Autodesk Inventor part; units mm, degrees
ref_plane "YZ Plane" through (0, 0, 0) normal (1, 0, 0) x (0, 1, 0)
ref_plane "XZ Plane" through (0, 0, 0) normal (0, 1, 0) x (-1, 0, 0)
ref_plane "XY Plane" through (0, 0, 0) normal (0, 0, 1) x (1, 0, 0)
sketch "Sketch1" plane through (0, 0, 0) normal (0, 1, 0) x (-1, 0, 0)
  line L0 (0, 0) -> (-111, 0)
  line L1 (-111, 0) -> (-111, -34)
  line L2 (-111, -34) -> (0, -34)
  line L3 (0, -34) -> (0, 0)
  dimension "d0" = 111
  dimension "d1" = 34
extrude "Extrusion1" add sketch "Sketch1" along normal blind 3.5
sketch "Sketch2" plane through (0, 3.5, 0) normal (0, 1, 0) x (1, 0, 0)
  line L0 (10, 9.825) -> (40, 9.825)
  line L1 (40, 9.825) -> (40, 24.175)
  line L2 (40, 24.175) -> (10, 24.175)
  line L3 (10, 24.175) -> (10, 9.825)
  line L4 (66.65, 9.825) -> (96.65, 9.825)
  line L5 (96.65, 9.825) -> (96.65, 24.175)
  line L6 (96.65, 24.175) -> (66.65, 24.175)
  line L7 (66.65, 24.175) -> (66.65, 9.825)
  point P0 (0, 0)
  point P1 (66.65, 17)
  dimension "d4" = 30
  dimension "d5" = 14.35
  dimension "d6" = 30
  dimension "d7" = 14.35
  dimension "d8" = 26.65
extrude "Extrusion2" cut sketch "Sketch2" against normal blind 3.5
fillet "Fillet1" radius 2 8 edges at (10, 1.75, -24.175) (40, 1.75, -24.175) (10, 1.75, -9.825) (40, 1.75, -9.825) (66.65, 1.75, -9.825) (66.65, 1.75, -24.175) (96.65, 1.75, -9.825) (96.65, 1.75, -24.175)
properties part number "arcade_lid_extrusion_3.5"
Can you work these out from the model? Positions are in its coordinate system, mm. A direction names the side the tool comes from. Give positions to 0.01 mm unless a question says otherwise; leave off trailing zeros. Loops run counter-clockwise (first coordinate to the right, second up) from the corner with the lowest first, then second, coordinate; pieces in that order, holes last. Notation, with made-up numbers: M 71.25,14.5 L 125.25,14.5 A5 ccw 125.25,21.5 Z; hole C 73.5,-23 d2. An arc over 180 degrees is marked long. One line per question, with ' | ' between items. Start each with the question number.
Q1. For faces 1 (the flat face through (56, 2, -34)), 2 (the cylindrical face through (67.251, 1.726, -10.395)), which set-ups out of +Z, -Z, +X, -X, +Y, -Y let a thin tool reach every point of the face, with its end or its side?
Q2. If I drill on line 1 (X direction, y = 1, z = -18.5); line 2 (Z direction, x = 90, y = 1.3) (3 decimals); line 3 (Z direction, x = 39.5, y = 0.8), over which ranges is the centre line in solid material (lowest first)? Write a range as from..to.
Q3. If we section it at A-A (x = 36.5): Please give me the cut outline in (y, z) (3 decimals), plus the area to 3 significant figures.
Q4. If we section it at C-C (y = 2): Please give me the cut outline in (x, z) (3 decimals), plus the area to 3 significant figures.
Q5. If we mould it in two halves opening along X, with no side actions, what happens to faces 3 (the flat face through (0, 2, -17)), 4 (the cylindrical face through (10.57, 1.726, -23.574)), 5 (the flat face through (55, 2, 0))? For each: +X half, -X half, draft (parallel to the pull), parting line (faces both ways), or undercut.
Q6. If we section it at B-B (z = -17): Please give me the cut outline in (x, y), plus the area to 4 significant figures.
Computed:
1) face 1: -Z, +X, -X, +Y, -Y | face 2: +Y, -Y
2) line 1: x = 0..10, 40..66.65, 96.65..111 | line 2: z = -34..-24.175, -9.825..0 | line 3: z = -34..-23.5, -10.5..0
3) outline: M 0,-34 L 3.5,-34 L 3.5,-24.175 L 0,-24.175 Z; M 0,-9.825 L 3.5,-9.825 L 3.5,0 L 0,0 Z | area: 68.8 mm²
4) outline: M 0,-34 L 111,-34 L 111,0 L 0,0 Z; hole M 10,-22.175 A2 ccw 12,-24.175 L 38,-24.175 A2 ccw 40,-22.175 L 40,-11.825 A2 ccw 38,-9.825 L 12,-9.825 A2 ccw 10,-11.825 Z; hole M 66.65,-22.175 A2 ccw 68.65,-24.175 L 94.65,-24.175 A2 ccw 96.65,-22.175 L 96.65,-11.825 A2 ccw 94.65,-9.825 L 68.65,-9.825 A2 ccw 66.65,-11.825 Z | area: 2,920 mm²
5) face 3: -X half | face 4: undercut | face 5: draft
6) outline: M 0,0 L 10,0 L 10,3.5 L 0,3.5 Z; M 40,0 L 66.65,0 L 66.65,3.5 L 40,3.5 Z; M 96.65,0 L 111,0 L 111,3.5 L 96.65,3.5 Z | area: 178.5 mm²
